from build123d import *

# Parameters (mm, degrees)
SKETCH1_W           = 190.5
SKETCH1_H           = 25.4
BOSS_EXTRUDE3_DEPTH = 1.64
SKETCH1_9_R         = 2.11
CUT_EXTRUDE8_DEPTH  = 1.64


with BuildPart() as part:
    # Sketch1 → Boss-Extrude3 (new body)
    with BuildSketch(Plane.XY):
        with Locations((-58.027959696, 19.972489638)):
            Rectangle(SKETCH1_W, SKETCH1_H)
    extrude(amount=BOSS_EXTRUDE3_DEPTH)

    # Sketch1_9 → Cut-Extrude8 (cut)
    with BuildSketch(Plane.XY):
        with BuildLine():
            Line((3.876326018, 27.962489638), (3.876326018, 23.662489638))
            ThreePointArc((3.876326018, 23.662489638), (5.986326018, 21.552489638), (8.096326018, 23.662489638))
            Line((8.096326018, 23.662489638), (8.096326018, 27.962489638))
            ThreePointArc((8.096326018, 27.962489638), (5.986326018, 30.072489638), (3.876326018, 27.962489638))
        make_face()
        with BuildLine():
            Line((-8.926531125, 27.962489638), (-8.926531125, 23.662489638))
            ThreePointArc((-8.926531125, 23.662489638), (-6.816531125, 21.552489638), (-4.706531125, 23.662489638))
            Line((-4.706531125, 23.662489638), (-4.706531125, 27.962489638))
            ThreePointArc((-4.706531125, 27.962489638), (-6.816531125, 30.072489638), (-8.926531125, 27.962489638))
        make_face()
        with BuildLine():
            Line((-21.729388268, 27.962489638), (-21.729388268, 23.662489638))
            ThreePointArc((-21.729388268, 23.662489638), (-19.619388268, 21.552489638), (-17.509388268, 23.662489638))
            Line((-17.509388268, 23.662489638), (-17.509388268, 27.962489638))
            ThreePointArc((-17.509388268, 27.962489638), (-19.619388268, 30.072489638), (-21.729388268, 27.962489638))
        make_face()
        with BuildLine():
            Line((-34.532245411, 27.962489638), (-34.532245411, 23.662489638))
            ThreePointArc((-34.532245411, 23.662489638), (-32.422245411, 21.552489638), (-30.312245411, 23.662489638))
            Line((-30.312245411, 23.662489638), (-30.312245411, 27.962489638))
            ThreePointArc((-30.312245411, 27.962489638), (-32.422245411, 30.072489638), (-34.532245411, 27.962489638))
        make_face()
        with BuildLine():
            Line((-47.335102553, 27.962489638), (-47.335102553, 23.662489638))
            ThreePointArc((-47.335102553, 23.662489638), (-45.225102553, 21.552489638), (-43.115102553, 23.662489638))
            Line((-43.115102553, 23.662489638), (-43.115102553, 27.962489638))
            ThreePointArc((-43.115102553, 27.962489638), (-45.225102553, 30.072489638), (-47.335102553, 27.962489638))
        make_face()
        with BuildLine():
            Line((-72.940816839, 27.962489638), (-72.940816839, 23.662489638))
            ThreePointArc((-72.940816839, 23.662489638), (-70.830816839, 21.552489638), (-68.720816839, 23.662489638))
            Line((-68.720816839, 23.662489638), (-68.720816839, 27.962489638))
            ThreePointArc((-68.720816839, 27.962489638), (-70.830816839, 30.072489638), (-72.940816839, 27.962489638))
        make_face()
        with Locations((31.592040304, 13.742489638)):
            Circle(SKETCH1_9_R)
        with Locations((18.789183161, 13.742489638)):
            Circle(SKETCH1_9_R)
        with Locations((5.986326018, 13.742489638)):
            Circle(SKETCH1_9_R)
        with Locations((-6.816531125, 13.742489638)):
            Circle(SKETCH1_9_R)
        with Locations((-19.619388268, 13.742489638)):
            Circle(SKETCH1_9_R)
        with Locations((-32.422245411, 13.742489638)):
            Circle(SKETCH1_9_R)
        with Locations((-45.225102553, 13.742489638)):
            Circle(SKETCH1_9_R)
        with Locations((-70.830816839, 13.742489638)):
            Circle(SKETCH1_9_R)
        with Locations((-83.633673982, 13.742489638)):
            Circle(SKETCH1_9_R)
        with Locations((-109.239388268, 13.742489638)):
            Circle(SKETCH1_9_R)
        with BuildLine():
            Line((-98.546531125, 27.962489638), (-98.546531125, 23.662489638))
            ThreePointArc((-98.546531125, 23.662489638), (-96.436531125, 21.552489638), (-94.326531125, 23.662489638))
            Line((-94.326531125, 23.662489638), (-94.326531125, 27.962489638))
            ThreePointArc((-94.326531125, 27.962489638), (-96.436531125, 30.072489638), (-98.546531125, 27.962489638))
        make_face()
        with BuildLine():
            Line((-85.743673982, 27.962489638), (-85.743673982, 23.662489638))
            ThreePointArc((-85.743673982, 23.662489638), (-83.633673982, 21.552489638), (-81.523673982, 23.662489638))
            Line((-81.523673982, 23.662489638), (-81.523673982, 27.962489638))
            ThreePointArc((-81.523673982, 27.962489638), (-83.633673982, 30.072489638), (-85.743673982, 27.962489638))
        make_face()
        with Locations((-122.042245411, 13.742489638)):
            Circle(SKETCH1_9_R)
        with BuildLine():
            Line((-136.955102553, 27.962489638), (-136.955102553, 23.662489638))
            ThreePointArc((-136.955102553, 23.662489638), (-134.845102553, 21.552489638), (-132.735102553, 23.662489638))
            Line((-132.735102553, 23.662489638), (-132.735102553, 27.962489638))
            ThreePointArc((-132.735102553, 27.962489638), (-134.845102553, 30.072489638), (-136.955102553, 27.962489638))
        make_face()
        with Locations((-134.845102553, 13.742489638)):
            Circle(SKETCH1_9_R)
        with BuildLine():
            Line((-149.757959696, 27.962489638), (-149.757959696, 23.662489638))
            ThreePointArc((-149.757959696, 23.662489638), (-147.647959696, 21.552489638), (-145.537959696, 23.662489638))
            Line((-145.537959696, 23.662489638), (-145.537959696, 27.962489638))
            ThreePointArc((-145.537959696, 27.962489638), (-147.647959696, 30.072489638), (-149.757959696, 27.962489638))
        make_face()
        with Locations((-147.647959696, 13.742489638)):
            Circle(SKETCH1_9_R)
        with BuildLine():
            Line((33.702040304, 27.962489638), (33.702040304, 23.662489638))
            ThreePointArc((33.702040304, 23.662489638), (31.592040304, 21.552489638), (29.482040304, 23.662489638))
            Line((29.482040304, 23.662489638), (29.482040304, 27.962489638))
            ThreePointArc((29.482040304, 27.962489638), (31.592040304, 30.072489638), (33.702040304, 27.962489638))
        make_face()
        with BuildLine():
            Line((20.899183161, 27.962489638), (20.899183161, 23.662489638))
            ThreePointArc((20.899183161, 23.662489638), (18.789183161, 21.552489638), (16.679183161, 23.662489638))
            Line((16.679183161, 23.662489638), (16.679183161, 27.962489638))
            ThreePointArc((16.679183161, 27.962489638), (18.789183161, 30.072489638), (20.899183161, 27.962489638))
        make_face()
        with BuildLine():
            Line((-55.917959696, 27.962489638), (-55.917959696, 23.662489638))
            ThreePointArc((-55.917959696, 23.662489638), (-58.027959696, 21.552489638), (-60.137959696, 23.662489638))
            Line((-60.137959696, 23.662489638), (-60.137959696, 27.962489638))
            ThreePointArc((-60.137959696, 27.962489638), (-58.027959696, 30.072489638), (-55.917959696, 27.962489638))
        make_face()
        with Locations((-58.027959696, 13.742489638)):
            Circle(SKETCH1_9_R)
        with Locations((-96.436531125, 13.742489638)):
            Circle(SKETCH1_9_R)
        with BuildLine():
            Line((-107.129388268, 27.962489638), (-107.129388268, 23.662489638))
            ThreePointArc((-107.129388268, 23.662489638), (-109.239388268, 21.552489638), (-111.349388268, 23.662489638))
            Line((-111.349388268, 23.662489638), (-111.349388268, 27.962489638))
            ThreePointArc((-111.349388268, 27.962489638), (-109.239388268, 30.072489638), (-107.129388268, 27.962489638))
        make_face()
        with BuildLine():
            Line((-119.932245411, 27.962489638), (-119.932245411, 23.662489638))
            ThreePointArc((-119.932245411, 23.662489638), (-122.042245411, 21.552489638), (-124.152245411, 23.662489638))
            Line((-124.152245411, 23.662489638), (-124.152245411, 27.962489638))
            ThreePointArc((-124.152245411, 27.962489638), (-122.042245411, 30.072489638), (-119.932245411, 27.962489638))
        make_face()
    extrude(amount=CUT_EXTRUDE8_DEPTH, mode=Mode.SUBTRACT)


solid = part.part
The model under review builds one solid part; all positions refer to its coordinate system, in mm. Coordinates: 2 decimals unless noted, no trailing zeros. Write each loop counter-clockwise with the first axis right and the second up, starting at its lowest first coordinate (ties: lowest second). Pieces come first, ordered by that corner, then holes. Notation, with made-up numbers: (58.25, 42) -> (93.25, 42) arc R26 ccw to (93.25, 64) -> close; hole circle Ø11 at (68.5, 67). An arc over 180 degrees is marked (long way). Answer in a Markdown table with one row per item.
1. We need section A-A, the plane x = -122. State the section outline as (y, z) points, and give its area (3 significant figures).
Answers below:
| item | result |
|---|---|
| outline | (7.27, 0) -> (11.63, 0) -> (11.63, 1.64) -> (7.27, 1.64) -> close; (15.85, 0) -> (21.55, 0) -> (21.55, 1.64) -> (15.85, 1.64) -> close; (30.07, 0) -> (32.67, 0) -> (32.67, 1.64) -> (30.07, 1.64) -> close |
| area | 20.8 mm^2 |
2. Clearance check with a flat-ended pin moving along its axis: pin 1 Ø4 at (x, y) = (-134.85, 13.74) entering from +Z. State where the tip first meets the part, or that it passes through.
Answers below:
| item | result |
|---|---|
| pin 1 | passes through |
3. Draft analysis for pull direction X (two halves, no side actions). For faces 1 (the cylindrical face through (-85.74, 13.84, 0.81)), 2 (the flat face through (-59, 20, 1.64)), state which applies: +X half, -X half, draft (parallel to the pull), parting line (faces both ways), or undercut.
Answers below:
| item | result |
|---|---|
| face 1 | undercut |
| face 2 | draft |
4. Wall thickness on probe 1 along Y at (x, z) = (-31, 0.7): over which ranges is the line inside the solid? List them lowest first. Write a range as [from, to].
Answers below:
| item | result |
|---|---|
| probe 1 | y = [7.27, 12.18], [15.3, 22.1], [29.52, 32.67] |
5. We need section C-C, the plane x = 5.5. State the section outline as (y, z) points, and give its area (3 significant figures).
Answers below:
| item | result |
|---|---|
| outline | (7.27, 0) -> (11.69, 0) -> (11.69, 1.64) -> (7.27, 1.64) -> close; (15.8, 0) -> (21.61, 0) -> (21.61, 1.64) -> (15.8, 1.64) -> close; (30.02, 0) -> (32.67, 0) -> (32.67, 1.64) -> (30.02, 1.64) -> close |
| area | 21.1 mm^2 |
6. We need section B-B, the plane z = 0.35. Give the number of separate pieces and of enclosed holes in the cut face, and give its area (3 significant figures).
Answers below:
| item | result |
|---|---|
| separate pieces | 1 |
| enclosed holes | 30 |
| area | 4,150 mm^2 |
